Verification items for the finished model (mm, model axes). A direction names the side the tool comes from. Coordinates: 2 decimals unless noted, no trailing zeros. Write each loop counter-clockwise with the first axis right and the second up, starting at its lowest first coordinate (ties: lowest second). Pieces come first, ordered by that corner, then holes. Notation, with made-up numbers: (-6.75, 2) - (1.25, 2) arc R18 ccw to (1.25, 26) - close; hole circle Ø3 at (31, 11). An arc over 180 degrees is marked (long way). Use one line per item in the form item = value. Start each with the question number.
(1) Sectioned sample at B-B (x = 19). Record the cut outline in (y, z), and give its area (3 significant figures).
(2) Mould release check, pull along X, two halves, no side actions. Record for faces 1 (the flat face through (0, 0, -34)), 2 (the cylindrical face through (-0.146, 0.783, -49.775)), 3 (the cylindrical face through (34.33, 0.78, 33.38)): released by +X, released by -X, zero draft, split by the parting line, or undercut.
(3) Material ranges on line 1 (Z direction, x = -4, y = 0.85); line 2 (X direction, y = 1.15, z = -0.5); line 3 (X direction, y = 0.95, z = -21), recorded low to high. Write a range as [from, to].
(4) Sectioned sample at A-A (z = -15). Record the cut outline in (x, y), and give its area (3 significant figures).
(5) Tool access check on faces 4 (the flat face through (0, 1.588, -34)), 5 (the cylindrical face through (26.67, 0.78, 25.88)). Record the directions out of +Z, -Z, +X, -X, +Y, -Y that give a thin tool (end or side, any length) a straight path to the whole face; none if there is none.
(6) Sectioned sample at C-C (y = 1.3). Count the separate pieces of the cut face and the enclosed holes in it, and give its area (3 significant figures).
(7) Gauge pin test, flat ends, axial feed: pin 1 Ø0.8 at (x, y) = (-40.5, 0.5) entering from -Z; pin 2 Ø5 at (x, z) = (-34.5, 33) entering from -Y; pin 3 Ø0.8 at (x, y) = (-1, 1) entering from +Z; pin 4 Ø0.6 at (y, z) = (0.5, -2) entering from +X. Record the tip position at first contact, or that the pin passes through.
from build123d import *

# Parameters (mm, degrees)
SKETCH1_R           = 3.71
SKETCH1_R_2         = 1.925
BOSS_EXTRUDE1_DEPTH = 1.5875
FILLET1_R           = 3
FILLET2_R           = 2
FILLET3_R           = 0.5


with BuildPart() as part:
    # Sketch1 → Boss-Extrude1 (new body)
    with BuildSketch(Plane(origin=(0, 0, 0), x_dir=(1, 0, 0), z_dir=(0, 1, 0))):
        with BuildLine():
            Line((-25.148871697, 32.027846467), (-0.825, 32.027846467))
            Line((-0.825, 32.027846467), (-0.825, 42.724341041))
            ThreePointArc((-0.825, 42.724341041), (0, 49.777846467), (0.825, 42.724341041))
            Line((0.825, 42.724341041), (0.825, 32.027846467))
            Line((0.825, 32.027846467), (25.148871697, 32.027846467))
            ThreePointArc((25.148871697, 32.027846467), (34.235092347, 34.992938814), (31.27, 25.906718164))
            Line((31.27, 25.906718164), (31.27, 1.582846467))
            Line((31.27, 1.582846467), (52.669827862, 1.582846467))
            Line((52.669827862, 1.582846467), (52.669827862, 2.092846467))
            Line((52.669827862, 2.092846467), (53.494827862, 2.092846467))
            Line((53.494827862, 2.092846467), (53.494827862, 1.582846467))
            Line((53.494827862, 1.582846467), (54.319827862, 1.582846467))
            Line((54.319827862, 1.582846467), (54.319827862, 2.092846467))
            Line((54.319827862, 2.092846467), (55.144827862, 2.092846467))
            Line((55.144827862, 2.092846467), (55.144827862, -0.577153533))
            Line((55.144827862, -0.577153533), (54.319827862, -0.577153533))
            Line((54.319827862, -0.577153533), (54.319827862, -0.067153533))
            Line((54.319827862, -0.067153533), (53.494827862, -0.067153533))
            Line((53.494827862, -0.067153533), (53.494827862, -0.577153533))
            Line((53.494827862, -0.577153533), (52.669827862, -0.577153533))
            Line((52.669827862, -0.577153533), (52.669827862, -0.067153533))
            Line((52.669827862, -0.067153533), (31.27, -0.067153533))
            Line((31.27, -0.067153533), (31.27, -24.39102523))
            ThreePointArc((31.27, -24.39102523), (34.235092347, -33.47724588), (25.148871697, -30.512153533))
            Line((25.148871697, -30.512153533), (0.825, -30.512153533))
            Line((0.825, -30.512153533), (0.825, -41.208648107))
            ThreePointArc((0.825, -41.208648107), (0, -48.262153533), (-0.825, -41.208648107))
            Line((-0.825, -41.208648107), (-0.825, -30.512153533))
            Line((-0.825, -30.512153533), (-25.148871697, -30.512153533))
            ThreePointArc((-25.148871697, -30.512153533), (-34.235092347, -33.47724588), (-31.27, -24.39102523))
            Line((-31.27, -24.39102523), (-31.27, -0.067153533))
            Line((-31.27, -0.067153533), (-52.669827862, -0.067153533))
            Line((-52.669827862, -0.067153533), (-52.669827862, -0.577153533))
            Line((-52.669827862, -0.577153533), (-53.494827862, -0.577153533))
            Line((-53.494827862, -0.577153533), (-53.494827862, -0.067153533))
            Line((-53.494827862, -0.067153533), (-54.319827862, -0.067153533))
            Line((-54.319827862, -0.067153533), (-54.319827862, -0.577153533))
            Line((-54.319827862, -0.577153533), (-55.144827862, -0.577153533))
            Line((-55.144827862, -0.577153533), (-55.144827862, 2.092846467))
            Line((-55.144827862, 2.092846467), (-54.319827862, 2.092846467))
            Line((-54.319827862, 2.092846467), (-54.319827862, 1.582846467))
            Line((-54.319827862, 1.582846467), (-53.494827862, 1.582846467))
            Line((-53.494827862, 1.582846467), (-53.494827862, 2.092846467))
            Line((-53.494827862, 2.092846467), (-52.669827862, 2.092846467))
            Line((-52.669827862, 2.092846467), (-52.669827862, 1.582846467))
            Line((-52.669827862, 1.582846467), (-31.27, 1.582846467))
            Line((-31.27, 1.582846467), (-31.27, 25.906718164))
            ThreePointArc((-31.27, 25.906718164), (-34.235092347, 34.992938814), (-25.148871697, 32.027846467))
        make_face()
        with Locations(Location((-30.445, 31.202846467, 0), (0, 0, 270))):
            Circle(SKETCH1_R, mode=Mode.SUBTRACT)
        with Locations(Location((30.445, 31.202846467, 0), (0, 0, 90))):
            Circle(SKETCH1_R, mode=Mode.SUBTRACT)
        with Locations(Location((30.445, -29.687153533, 0), (0, 0, 270))):
            Circle(SKETCH1_R, mode=Mode.SUBTRACT)
        with Locations(Location((-30.445, -29.687153533, 0), (0, 0, 90))):
            Circle(SKETCH1_R, mode=Mode.SUBTRACT)
        with Locations(Location((0, 46.202846467, 0), (0, 0, 270))):
            Circle(SKETCH1_R_2, mode=Mode.SUBTRACT)
        with Locations(Location((0, -44.687153533, 0), (0, 0, 90))):
            Circle(SKETCH1_R_2, mode=Mode.SUBTRACT)
        with BuildLine():
            Line((-25.148871697, 30.377846467), (25.148871697, 30.377846467))
            ThreePointArc((25.148871697, 30.377846467), (26.654907653, 27.41275412), (29.62, 25.906718164))
            Line((29.62, 25.906718164), (29.62, -24.39102523))
            ThreePointArc((29.62, -24.39102523), (26.654907653, -25.897061186), (25.148871697, -28.862153533))
            Line((25.148871697, -28.862153533), (-25.148871697, -28.862153533))
            ThreePointArc((-25.148871697, -28.862153533), (-26.654907653, -25.897061186), (-29.62, -24.39102523))
            Line((-29.62, -24.39102523), (-29.62, 25.906718164))
            ThreePointArc((-29.62, 25.906718164), (-26.654907653, 27.41275412), (-25.148871697, 30.377846467))
        make_face(mode=Mode.SUBTRACT)
    extrude(amount=BOSS_EXTRUDE1_DEPTH)

    # Fillet1
    fillet1_edges = [part.edges().sort_by_distance(p)[0] for p in [
        (-25.148871697, 0.79375, -30.377846467),
        (-29.62, 0.79375, -25.906718164),
        (-29.62, 0.79375, 24.39102523),
        (-25.148871697, 0.79375, 28.862153533),
        (25.148871697, 0.79375, 28.862153533),
        (29.62, 0.79375, 24.39102523),
        (29.62, 0.79375, -25.906718164),
        (25.148871697, 0.79375, -30.377846467),
        (31.27, 0.79375, 24.39102523),
        (25.148871697, 0.79375, 30.512153533),
        (-25.148871697, 0.79375, 30.512153533),
        (-31.27, 0.79375, 24.39102523),
        (-31.27, 0.79375, -25.906718164),
        (-25.148871697, 0.79375, -32.027846467),
        (25.148871697, 0.79375, -32.027846467),
        (31.27, 0.79375, -25.906718164),
    ]]
    fillet(fillet1_edges, radius=FILLET1_R)

    # Fillet2
    fillet2_edges = [part.edges().sort_by_distance(p)[0] for p in [
        (31.27, 0.79375, 0.067153533),
        (0.825, 0.79375, 30.512153533),
        (-0.825, 0.79375, 30.512153533),
        (-31.27, 0.79375, 0.067153533),
        (-31.27, 0.79375, -1.582846467),
        (-0.825, 0.79375, -32.027846467),
        (0.825, 0.79375, -32.027846467),
        (31.27, 0.79375, -1.582846467),
    ]]
    fillet(fillet2_edges, radius=FILLET2_R)

    # Fillet3
    fillet3_edges = [part.edges().sort_by_distance(p)[0] for p in [
        (55.144827862, 0.79375, -2.092846467),
        (55.144827862, 0.79375, 0.577153533),
        (-55.144827862, 0.79375, 0.577153533),
        (-55.144827862, 0.79375, -2.092846467),
    ]]
    fillet(fillet3_edges, radius=FILLET3_R)


solid = part.part
Answers below:
q1.outline = (0, -32.03) - (1.59, -32.03) - (1.59, -30.38) - (0, -30.38) - close; (0, 28.86) - (1.59, 28.86) - (1.59, 30.51) - (0, 30.51) - close
q1.area = 5.24 mm2
q2.face_1 = zero draft
q2.face_2 = split by the parting line
q2.face_3 = undercut
q3.line_1 = [-32.03, -30.38], [28.86, 30.51]
q3.line_2 = [-55.14, -29.62], [29.62, 55.14]
q3.line_3 = [-31.27, -29.62], [29.62, 31.27]
q4.outline = (-31.27, 0) - (-29.62, 0) - (-29.62, 1.59) - (-31.27, 1.59) - close; (29.62, 0) - (31.27, 0) - (31.27, 1.59) - (29.62, 1.59) - close
q4.area = 5.24 mm2
q5.face_4 = +Z, -Z, +X, -X, +Y
q5.face_5 = +Y, -Y
q6.separate_pieces = 1
q6.enclosed_holes = 7
q6.area = 712 mm2
q7.pin_1 = -1.58
q7.pin_2 = 0
q7.pin_3 = 48.21
q7.pin_4 = 55.13
